Geometry check sheet. Reference: the model listing, model coordinates, mm. A direction names the side the tool comes from. Give positions to 0.01 mm unless a question says otherwise; leave off trailing zeros. Order: outer loops, then holes, each group sorted by start corner. A loop starts at its lowest first (then second) coordinate and runs counter-clockwise, first axis right, second up. Notation, with made-up numbers: M 2.25,74.5 L 26.25,74.5 A15 ccw 26.25,78.5 Z; hole C 27,13 d7. An arc over 180 degrees is marked long. Answer as CSV lines item,"result". Start each with the question number.
Q1. Mould release check, pull along Y, two halves, no side actions. Record for faces 5 (the cylindrical face through (30.79, 71.5, 3.13)), 6 (the flat face through (57.15, 53, 3)), 7 (the flat face through (50.8, 33, 3)): +Y half, -Y half, draft (parallel to the pull), parting line (faces both ways), or undercut.
Q2. Go/stop test with flat-tipped pins: pin 1 (1.4 mm diameter, centred on y = 67, z = 4.5, fed in from +X); pin 2 (1 mm diameter, centred on y = 27.5, z = 3.5, fed in from +X); pin 3 (1.9 mm diameter, centred on y = 63.5, z = 3, fed in from -X). Record where each tip stops, or that it passes through.
Q3. Section check A-A, the plane z = 4.5. Record the boundary of the cut face in (x, y).
Q4. Section check B-B, the plane y = 62.5. Record the boundary of the cut face in (x, z), then the cut area to 3 significant figures.
Q5. Set-up check for faces 1 (the flat face through (54, 46.99, 3)), 2 (the flat face through (54, 59.69, 3)), 3 (the flat face through (18.923, 67, 3)), 4 (the flat face through (-3, 46.99, 3)): record each of +Z, -Z, +X, -X, +Y, -Y from which the full face is reachable in a straight line by a thin tool's end or side.
Q6. Thickness scan on line 1 (X direction, y = 25, z = 5.75); line 2 (Y direction, x = 18.5, z = 5.5); line 3 (X direction, y = 68.5, z = 4.25). Record the ranges inside material, lowest first.
```python
from build123d import *

# Parameters (mm, degrees)
SKETCH1_W           = 50.8
SKETCH1_H           = 66.04
BOSS_EXTRUDE1_DEPTH = 6.35
SKETCH2_W           = 6.35
SKETCH2_H           = 12.7
BOSS_EXTRUDE2_DEPTH = 6.35


with BuildPart() as part:
    # Sketch1 → Boss-Extrude1 (new body)
    with BuildSketch(Plane.XY):
        with Locations((25.4, 33.02)):
            Rectangle(SKETCH1_W, SKETCH1_H)
    extrude(amount=BOSS_EXTRUDE1_DEPTH)

    # Sketch2 → Boss-Extrude2 (add)
    with BuildSketch(Plane.XY):
        with Locations((-3.175, 53.34)):
            Rectangle(SKETCH2_W, SKETCH2_H)
        with Locations((-3.175, 12.7)):
            Rectangle(SKETCH2_W, SKETCH2_H)
        with Locations((53.975, 12.7)):
            Rectangle(SKETCH2_W, SKETCH2_H)
        with Locations((53.975, 53.34)):
            Rectangle(SKETCH2_W, SKETCH2_H)
        with BuildLine():
            Line((18.923, 66.04), (31.877, 66.04))
            Line((31.877, 66.04), (31.877, 68.834))
            ThreePointArc((31.877, 68.834), (30.761076836, 71.528076836), (28.067, 72.644))
            Line((28.067, 72.644), (22.733, 72.644))
            ThreePointArc((22.733, 72.644), (20.038923164, 71.528076836), (18.923, 68.834))
            Line((18.923, 68.834), (18.923, 66.04))
        make_face()
    extrude(amount=BOSS_EXTRUDE2_DEPTH)


solid = part.part
```
Answer block:
1,face 5,"+Y half"
1,face 6,"draft"
1,face 7,"undercut"
2,pin 1,"stops at x = 31.88"
2,pin 2,"stops at x = 50.8"
2,pin 3,"stops at x = 0"
3,outline,"M -6.35,6.35 L 0,6.35 L 0,0 L 50.8,0 L 50.8,6.35 L 57.15,6.35 L 57.15,19.05 L 50.8,19.05 L 50.8,46.99 L 57.15,46.99 L 57.15,59.69 L 50.8,59.69 L 50.8,66.04 L 31.88,66.04 L 31.88,68.83 A3.81 ccw 28.07,72.64 L 22.73,72.64 A3.81 ccw 18.92,68.83 L 18.92,66.04 L 0,66.04 L 0,59.69 L -6.35,59.69 L -6.35,46.99 L 0,46.99 L 0,19.05 L -6.35,19.05 Z"
4,outline,"M 0,0 L 50.8,0 L 50.8,6.35 L 0,6.35 Z"
4,area,"323 mm2"
5,face 1,"+Z, -Z, +X"
5,face 2,"+Z, -Z, +X, +Y"
5,face 3,"+Z, -Z, -X, +Y"
5,face 4,"+Z, -Z, -X"
6,line 1,"x = 0 to 50.8"
6,line 2,"y = 0 to 66.04"
6,line 3,"x = 18.92 to 31.88"
